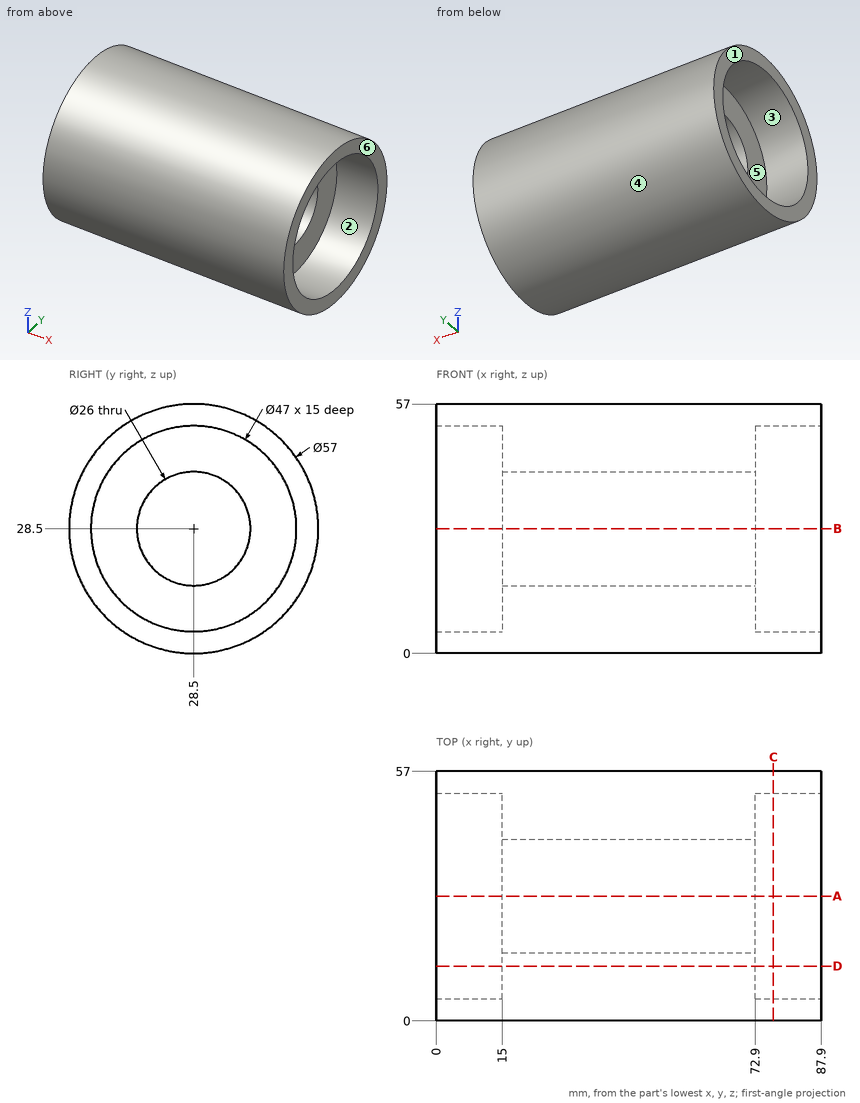
The figure shows three views and two pictorial views of one solid part (mm, origin at its lowest corner). Answer the questions. A direction names the side the tool comes from. Coordinates: 2 decimals unless noted, no trailing zeros. Loops run counter-clockwise (first coordinate to the right, second up) from the corner with the lowest first, then second, coordinate; pieces in that order, holes last. Notation, with made-up numbers: M -40,42 L -21,42 A12 ccw -21,57 Z; hole C -32.75,24.5 d3. An arc over 180 degrees is marked long. Use CSV: the item, a comma, the result in double quotes. Start each with the question number.
(1) Find section C-C, the plane x = 77. Give the vertices of the cut face in (y, z).
(2) Find section A-A, the plane y = 28.5. Give the vertices of the cut face in (x, z), then the cut area to 3 significant figures.
(3) Consider line 1 (Y direction, x = 10.25, z = 28.5); line 2 (X direction, y = 11, z = 44); line 3 (Z direction, x = 85, y = 28). Determine where each line is inside the solid, lowest interval first.
(4) Find section D-D, the plane y = 12.5. Give the vertices of the cut face in (x, z).
(5) Given pin 1 Ø6 at (y, z) = (46.5, 17.5) entering from +X; pin 2 Ø8 at (y, z) = (19.5, 18) entering from -X; pin 3 Ø10 at (x, y) = (10, 35.5) entering from -Z; pin 4 Ø1 at (x, y) = (66, 32) entering from -Z, each flat-ended and moving along its own axis, determine where each tip first touches the part or whether it passes through.
(6) For a pull along Y with two mould halves and no side action, classify the marked faces 4, 5 and 6 as +Y half, -Y half, draft (parallel to the pull), parting line (faces both ways), or undercut.
(7) For the marked faces 1, 2 and 3, determine the directions among +Z, -Z, +X, -X, +Y, -Y from which every point of the face is accessible in a straight line to the end or side of a thin tool.
Recorded:
1,outline,"C 28.5,28.5 d57; hole C 28.5,28.5 d47"
2,outline,"M 0,0 L 87.9,0 L 87.9,5 L 72.9,5 L 72.9,15.5 L 15,15.5 L 15,5 L 0,5 Z; M 0,52 L 15,52 L 15,41.5 L 72.9,41.5 L 72.9,52 L 87.9,52 L 87.9,57 L 0,57 Z"
2,area,"2,090 mm^2"
3,line 1,"y = 0 to 5, 52 to 57"
3,line 2,"x = 15 to 72.9"
3,line 3,"z = 0 to 5.01, 51.99 to 57"
4,outline,"M 0,4.92 L 87.9,4.92 L 87.9,11.29 L 72.9,11.29 L 72.9,45.71 L 87.9,45.71 L 87.9,52.08 L 0,52.08 L 0,45.71 L 15,45.71 L 15,11.29 L 0,11.29 Z"
5,pin 1,"stops at x = 87.9"
5,pin 2,"stops at x = 15"
5,pin 3,"stops at z = 0.07"
5,pin 4,"stops at z = 0.16"
6,face 4,"parting line"
6,face 5,"undercut"
6,face 6,"draft"
7,face 1,"+Z, -Z, -X, +Y, -Y"
7,face 2,"+X"
7,face 3,"-X"
